from build123d import *

# Parameters (mm, degrees)
F0_W     = 11.1125013079
F0_H     = 11.1125
F0_W_2   = 3.1749973842
F0_H_2   = 139.7
F0_W_3   = 88.9
F0_H_3   = 3.175
F1_DEPTH = 3.175
F2_DEPTH = 5.1418882795
F3_R     = 10.16


# Not quite as in the source:
# - ends of sketch curves that miss each other by under 0.0002 mm in the source are joined


with BuildPart() as f1:
    # F0 (on Top) → F1 (new body)
    with BuildSketch(Plane.XY):
        with Locations((-7.143749346, 7.14375)):
            Rectangle(F0_W, F0_H)
        with Locations((7.143749346, 7.14375)):
            Rectangle(F0_W, F0_H)
        with Locations((7.143749346, -7.14375)):
            Rectangle(F0_W, F0_H)
        with Locations((-7.143749346, -7.14375)):
            Rectangle(F0_W, F0_H)
        with Locations((0, 82.55)):
            Rectangle(F0_W_2, F0_H_2)
        Polygon((0, 1.5875), (1.5874986921, 1.5875), (1.5874986921, 12.7), (-1.5874986921, 12.7), (-1.5874986921, 1.5875), align=None)
        Polygon((1.5874986921, -1.5875), (12.7, -1.5875), (12.7, 1.5875), (1.5874986921, 1.5875), (1.5874986921, 0), align=None)
        Polygon((-12.7, -1.5875), (-1.5874986921, -1.5875), (-1.5874986921, 0), (-1.5874986921, 1.5875), (-12.7, 1.5875), align=None)
        Polygon((1.5874986921, -12.7), (1.5874986921, -1.5875), (0, -1.5875), (-1.5874986921, -1.5875), (-1.5874986921, -12.7), align=None)
        with Locations((0, -82.55)):
            Rectangle(F0_W_2, F0_H_2)
        with Locations((-57.15, 0)):
            Rectangle(F0_W_3, F0_H_3)
        with Locations((57.15, 0)):
            Rectangle(F0_W_3, F0_H_3)
        with BuildLine():
            Line((-1.5874986921, 1.5875), (-1.5874986921, 0))
            ThreePointArc((-1.5874986921, 0), (-1.1225320151, 1.1225320151), (0, 1.5875))
            Line((0, 1.5875), (-1.5874986921, 1.5875))
        make_face()
        with BuildLine():
            ThreePointArc((-1.5875, 0), (-1.1225320151, -1.1225320151), (0, -1.5875))
            ThreePointArc((0, -1.5875), (1.1225320151, -1.1225320151), (1.5875, 0))
            ThreePointArc((1.5875, 0), (1.1225320151, 1.1225320151), (0, 1.5875))
            ThreePointArc((0, 1.5875), (-1.1225320151, 1.1225320151), (-1.5875, 0))
        make_face()
        with BuildLine():
            ThreePointArc((0, 1.5875), (1.1225320151, 1.1225320151), (1.5875, 0))
            Line((1.5875, 0), (1.5874986921, 1.5875))
            Line((1.5874986921, 1.5875), (0, 1.5875))
        make_face()
        with BuildLine():
            Line((-1.5874986921, -1.5875), (0, -1.5875))
            ThreePointArc((0, -1.5875), (-1.1225320151, -1.1225320151), (-1.5875, 0))
            Line((-1.5875, 0), (-1.5874986921, -1.5875))
        make_face()
        with BuildLine():
            Line((0, -1.5875), (1.5874986921, -1.5875))
            Line((1.5874986921, -1.5875), (1.5874986921, 0))
            ThreePointArc((1.5874986921, 0), (1.1225320151, -1.1225320151), (0, -1.5875))
        make_face()
    extrude(amount=F1_DEPTH)

    # F0 (on Top) → F2 (join)
    with BuildSketch(Plane.XY):
        with BuildLine():
            ThreePointArc((-1.5875, 0), (-1.1225320151, -1.1225320151), (0, -1.5875))
            ThreePointArc((0, -1.5875), (1.1225320151, -1.1225320151), (1.5875, 0))
            ThreePointArc((1.5875, 0), (1.1225320151, 1.1225320151), (0, 1.5875))
            ThreePointArc((0, 1.5875), (-1.1225320151, 1.1225320151), (-1.5875, 0))
        make_face()
    extrude(amount=F2_DEPTH)

    # F3
    f3_edges = [f1.edges().sort_by_distance(p)[0] for p in [
        (12.7, -12.7, 1.5875),
        (-12.7, -12.7, 1.5875),
        (12.7, 12.7, 1.5875),
        (-12.7, 12.7, 1.5875),
    ]]
    fillet(f3_edges, radius=F3_R)


solid = f1.part
Verification items for the finished model (mm, model axes). A direction names the side the tool comes from. Coordinates: 2 decimals unless noted, no trailing zeros. Write each loop counter-clockwise with the first axis right and the second up, starting at its lowest first coordinate (ties: lowest second). Pieces come first, ordered by that corner, then holes. Notation, with made-up numbers: M 9.25,76 L 35.25,76 A28 ccw 35.25,101 Z; hole C 34.25,59.5 d11. An arc over 180 degrees is marked long. Use a Markdown table: item, result.
Q1. Sectioned sample at B-B, the plane y = 93. Record the boundary of the cut face in (x, z) (1 decimal), plus the area to 3 significant figures.
Reply:
| item | result |
|---|---|
| outline | M -1.6,0 L 1.6,0 L 1.6,3.2 L -1.6,3.2 Z |
| area | 10.1 mm² |
Q2. Set-up check for faces 1 (the face through (-9.803, 9.645, 1.61)), 2 (the face through (-8, 1, 3.175)): record each of +Z, -Z, +X, -X, +Y, -Y from which the full face is reachable in a straight line by a thin tool's end or side.
Reply:
| item | result |
|---|---|
| face 1 | +Z, -Z, -X, +Y |
| face 2 | +Z |
Q3. Go/stop test with flat-tipped pins: P1, Ø2.5, axis at y = -86.5, z = 1, coming from the +X side; P2, Ø1, axis at y = -82.5, z = 2.5, coming from the -X side; P3, Ø2.5, axis at x = -76.5, z = 2, coming from the +Y side; P4, Ø1, axis at x = -24.5, z = 4, coming from the -Y side. Record where each tip stops, or that it passes through.
Reply:
| item | result |
|---|---|
| P1 | stops at x = 1.59 |
| P2 | stops at x = -1.59 |
| P3 | stops at y = 1.59 |
| P4 | passes through |
Q4. Sectioned sample at A-A, the plane z = 2. Record the boundary of the cut face in (x, y).
Reply:
| item | result |
|---|---|
| outline | M -101.6,-1.59 L -12.7,-1.59 L -12.7,-2.54 A10.16 ccw -2.54,-12.7 L -1.59,-12.7 L -1.59,-152.4 L 1.59,-152.4 L 1.59,-12.7 L 2.54,-12.7 A10.16 ccw 12.7,-2.54 L 12.7,-1.59 L 101.6,-1.59 L 101.6,1.59 L 12.7,1.59 L 12.7,2.54 A10.16 ccw 2.54,12.7 L 1.59,12.7 L 1.59,152.4 L -1.59,152.4 L -1.59,12.7 L -2.54,12.7 A10.16 ccw -12.7,2.54 L -12.7,1.59 L -101.6,1.59 Z |
Q5. Thickness scan on line 1 (X direction, y = 111, z = 2.6); line 2 (Z direction, x = -0.5, y = -99) (3 decimals). Record the ranges inside material, lowest first.
Reply:
| item | result |
|---|---|
| line 1 | x = -1.59 to 1.59 |
| line 2 | z = 0 to 3.175 |
